Verification items for the finished model (mm, model axes). A direction names the side the tool comes from. Round coordinates to 2 decimals unless told otherwise and drop trailing zeros. Loops run counter-clockwise (first coordinate to the right, second up) from the corner with the lowest first, then second, coordinate; pieces in that order, holes last. Notation, with made-up numbers: M -0.75,23 L 7.25,23 A29 cw 7.25,45 Z; hole C 71,23 d1. An arc over 180 degrees is marked long. Write item = value, one per line. Start each with the question number.
Autodesk Inventor part; units mm, degrees
ref_plane "YZ Plane" through (0, 0, 0) normal (1, 0, 0) x (0, 1, 0)
ref_plane "XZ Plane" through (0, 0, 0) normal (0, 1, 0) x (-1, 0, 0)
ref_plane "XY Plane" through (0, 0, 0) normal (0, 0, 1) x (1, 0, 0)
sketch "Sketch1" plane through (0, 0, 0) normal (1, 0, 0) x (0, 1, 0)
  circle A0 centre (11.54, 17.0818) radius 8.25
  point P0 (0, 0)
  dimension "d0" = 16.5
extrude "Plate1" add sketch "Sketch1" along normal blind 25.5
sketch "Sketch2" plane through (25.5, 11.54, 17.0818) normal (1, 0, 0) x (0, 0, -1)
  circle A0 centre (0, 0) radius 6.095
  point P0 (17.0818, -11.54)
  dimension "d2" = 12.19
extrude "Extrusion1" add sketch "Sketch2" along normal blind 5
sketch "Sketch3" plane through (30.5, 11.54, 17.0818) normal (1, 0, 0) x (0, 0, -1)
  circle A0 centre (0, 0) radius 3
  point P0 (17.0818, -11.54)
  dimension "d5" = 6
extrude "Extrusion2" add sketch "Sketch3" along normal blind 20
equation "\"d1\" = Thickness"
equation "\"BendRadius\" = Thickness"
equation "\"BendReliefWidth\" = Thickness"
equation "\"BendReliefDepth\" = 0.5 * Thickness"
equation "\"CornerReliefSize\" = 4 * Thickness"
equation "\"MinimumRemnant\" = 2 * Thickness"
equation "\"TransitionRadius\" = BendRadius"
equation "\"JacobiRadiusSize\" = BendRadius"
equation "\"GapSize\" = Thickness"
properties part number "dccc"
1. Section check D-D, the plane y = 6.25. Enter the section's corners in (x, z).
2. Thickness scan on line 1 (Z direction, x = 19.5, y = 11.75); line 2 (X direction, y = 10.5, z = 11); line 3 (Y direction, x = 11, z = 17.5). Record the ranges inside material, lowest first.
3. Section check C-C, the plane x = 34.5. Enter the section's corners in (y, z), and give its area (3 significant figures).
4. Section check B-B, the plane z = 22.5. Enter the section's corners in (x, y).
5. Gauge pin test, flat ends, axial feed: P1, Ø8, axis at x = 13.5, y = 6.5, coming from the +Z side; P2, Ø4, axis at x = 40.5, y = 15.5, coming from the -Z side; P3, Ø4, axis at x = 12.5, y = 16.5, coming from the +Z side. Record the tip position at first contact, or that the pin passes through.
6. Section check A-A, the plane y = 11.54. Enter the section's corners in (x, z).
7. Tool access check on faces 1 (the flat face through (50.5, 12, 17)), 2 (the cylindrical face through (40.36, 12.69, 14.31)). Record the directions out of +Z, -Z, +X, -X, +Y, -Y that give a thin tool (end or side, any length) a straight path to the whole face; none if there is none.
Computed values:
q1.outline = M 0,10.75 L 25.5,10.75 L 25.5,14.05 L 30.5,14.05 L 30.5,20.11 L 25.5,20.11 L 25.5,23.41 L 0,23.41 Z
q2.line_1 = 8.83 to 25.33
q2.line_2 = 0 to 25.5
q2.line_3 = 3.3 to 19.78
q3.outline = C 11.54,17.08 d6
q3.area = 28.3 mm2
q4.outline = M 0,5.32 L 25.5,5.32 L 25.5,8.75 L 30.5,8.75 L 30.5,14.33 L 25.5,14.33 L 25.5,17.76 L 0,17.76 Z
q5.P1 = 25.27
q5.P2 = 14.81
q5.P3 = 24.78
q6.outline = M 0,8.83 L 25.5,8.83 L 25.5,10.99 L 30.5,10.99 L 30.5,14.08 L 50.5,14.08 L 50.5,20.08 L 30.5,20.08 L 30.5,23.18 L 25.5,23.18 L 25.5,25.33 L 0,25.33 Z
q7.face_1 = +Z, -Z, +X, +Y, -Y
q7.face_2 = +X
